The listing builds one solid part. Answer for the finished solid, in the listing's coordinates (mm). A direction names the side the tool comes from. Coordinates: 2 decimals unless noted, no trailing zeros. Write each loop counter-clockwise with the first axis right and the second up, starting at its lowest first coordinate (ties: lowest second). Pieces come first, ordered by that corner, then holes.
from build123d import *

# Parameters (mm, degrees)
SKETCH001_R      = 9
EXTRUDE001_DEPTH = 4.5
SKETCH002_R      = 9.5
EXTRUDE002_DEPTH = 3.5
SKETCH003_R      = 11
EXTRUDE003_DEPTH = 2.5
SKETCH004_R      = 12
EXTRUDE004_DEPTH = 1.5
SKETCH_R         = 7.5
EXTRUDE_DEPTH    = 6


with BuildPart() as extrude001:
    # Sketch001 → Extrude001 (new body)
    with BuildSketch(Plane.XY):
        Circle(SKETCH001_R)
    extrude(amount=EXTRUDE001_DEPTH)


with BuildPart() as extrude002:
    # Sketch002 → Extrude002 (new body)
    with BuildSketch(Plane.XY):
        Circle(SKETCH002_R)
    extrude(amount=EXTRUDE002_DEPTH)


with BuildPart() as extrude003:
    # Sketch003 → Extrude003 (new body)
    with BuildSketch(Plane.XY):
        Circle(SKETCH003_R)
    extrude(amount=EXTRUDE003_DEPTH)


with BuildPart() as extrude004:
    # Sketch004 → Extrude004 (new body)
    with BuildSketch(Plane.XY):
        Circle(SKETCH004_R)
    extrude(amount=EXTRUDE004_DEPTH)


with BuildPart() as fusion:
    # Sketch → Extrude (new body)
    with BuildSketch(Plane.XY):
        Circle(SKETCH_R)
    extrude(amount=EXTRUDE_DEPTH)

    # Fusion: union Extrude001, Extrude002, Extrude003, Extrude004
    add(extrude001.part)
    add(extrude002.part)
    add(extrude003.part)
    add(extrude004.part)


solid = fusion.part
Q1. The part is cut by section C-C, the plane z = 5.55. Write down the section's boundary in (x, y).
Answers below:
outline: circle Ø15 at (0, 0)
Q2. Find the intervals of material crossed by probe 1 along Z at (x, y) = (6.25, -7.75); probe 2 along Z at (x, y) = (7.5, -2); probe 3 along Y at (x, z) = (2.5, 5.7), in increasing order.
Answers below:
probe 1: z = 0 to 2.5
probe 2: z = 0 to 4.5
probe 3: y = -7.07 to 7.07
Q3. Given pin 1 (3 mm diameter, centred on y = 6, z = 5, fed in from +X); pin 2 (2 mm diameter, centred on x = 8, y = 9, fed in from +Z); pin 3 (3 mm diameter, centred on x = 7, y = -7, fed in from +Z), each flat-ended and moving along its own axis, determine where each tip first touches the part or whether it passes through.
Answers below:
pin 1: stops at x = 7.74
pin 2: stops at z = 1.5
pin 3: stops at z = 4.5
Q4. The part is cut by section D-D, the plane x = -10. Write down the section's boundary in (y, z).
Answers below:
outline: (-6.63, 0) - (6.63, 0) - (6.63, 1.5) - (4.58, 1.5) - (4.58, 2.5) - (-4.58, 2.5) - (-4.58, 1.5) - (-6.63, 1.5) - close
Q5. The part is cut by section A-A, the plane y = 0. Write down the section's boundary in (x, z).
Answers below:
outline: (-12, 0) - (12, 0) - (12, 1.5) - (11, 1.5) - (11, 2.5) - (9.5, 2.5) - (9.5, 3.5) - (9, 3.5) - (9, 4.5) - (7.5, 4.5) - (7.5, 6) - (-7.5, 6) - (-7.5, 4.5) - (-9, 4.5) - (-9, 3.5) - (-9.5, 3.5) - (-9.5, 2.5) - (-11, 2.5) - (-11, 1.5) - (-12, 1.5) - close
Q6. Which of the six approach directions +Z, -Z, +X, -X, +Y, -Y give full straight-line access (tool end or side, diameter ignored) to faces 1 (the face through (-2.38, -10.74, 1.99)), 2 (the face through (0, 0, 0))?
Answers below:
face 1: +Z
face 2: -Z, +X, -X, +Y, -Y
